from build123d import *

# Parameters (mm, degrees)
BOSS_EXTRUDE1_DEPTH = 5
SKETCH2_R           = 1.5
BOSS_EXTRUDE2_DEPTH = 7
SKETCH4_R           = 1
CUT_EXTRUDE1_DEPTH  = 21.732622043


with BuildPart() as part:
    # Sketch1 → Boss-Extrude1 (new body)
    with BuildSketch(Plane.XY):
        with BuildLine():
            ThreePointArc((12.735353306, 10.993667304), (8.407166921, 10.537476108), (5.016332041, 7.809189722))
            ThreePointArc((5.016332041, 7.809189722), (3.545099052, 3.440082341), (7.125107355, 6.34476242))
            ThreePointArc((7.125107355, 6.34476242), (9.612326684, 9.052857395), (12.735353306, 10.993667304))
        make_face()
    extrude(amount=BOSS_EXTRUDE1_DEPTH)

    # Sketch2 → Boss-Extrude2 (add)
    with BuildSketch(Plane.XY.offset(5)):
        with Locations((4.914048995, 5.411370258)):
            Circle(SKETCH2_R)
    extrude(amount=BOSS_EXTRUDE2_DEPTH)

    # Sketch4 → Cut-Extrude1 (cut, through all)
    with BuildSketch(Plane(origin=(0, 0, 0), x_dir=(-1, 0, 0), z_dir=(0, 0, -1))):
        with Locations((-6.764513076, 8.009147455)):
            Circle(SKETCH4_R)
    extrude(amount=-CUT_EXTRUDE1_DEPTH, mode=Mode.SUBTRACT)


solid = part.part
Part model, mm, in its own coordinate system. A direction names the side the tool comes from. Coordinates: 2 decimals unless noted, no trailing zeros. Order: outer loops, then holes, each group sorted by start corner. A loop starts at its lowest first (then second) coordinate and runs counter-clockwise, first axis right, second up. Notation, with made-up numbers: M -13,41 L 45,41 A34 cw 45,71 Z; hole C 14.25,82 d9. An arc over 180 degrees is marked long. Use a Markdown table: item, result.
(1) Pull direction Y, two halves, no side cores. Call faces 1 (the cylindrical face through (8.46, 10.56, 2.46)), 2 (the flat face through (6, 7, 0)), 3 (the cylindrical face through (6.303, 7.122, 2.465)): released by +Y, released by -Y, zero draft, split by the parting line, or undercut.
A:
| item | result |
|---|---|
| face 1 | released by +Y |
| face 2 | zero draft |
| face 3 | undercut |
(2) Probe L1, parallel to Z at x = 6.5, y = 6.5; L2, parallel to Y at x = 6, z = 3.5; L3, parallel to Y at x = 10, z = 2.5. List the from-to ranges inside material, lowest first.
A:
| item | result |
|---|---|
| L1 | z = 0 to 5 |
| L2 | y = 3.27 to 7.36, 8.65 to 8.96 |
| L3 | y = 9.36 to 11 |
(3) Cut at A-A on x = 7.5. Write the cut outline in (y, z).
A:
| item | result |
|---|---|
| outline | M 6.86,0 L 7.33,0 L 7.33,5 L 6.86,5 Z; M 8.69,0 L 10.09,0 L 10.09,5 L 8.69,5 Z |
(4) Cut at C-C on y = 5.75. Write the cut outline in (x, z).
A:
| item | result |
|---|---|
| outline | M 2.54,0 L 7.29,0 L 7.29,5 L 6.38,5 L 6.38,12 L 3.45,12 L 3.45,5 L 2.54,5 Z |
(5) Cut at D-D on z = 2. Write the cut outline in (x, y).
A:
| item | result |
|---|---|
| outline | M 5.02,7.81 A2.4 ccw long 7.13,6.34 A13.57 cw 12.74,10.99 A7.71 ccw Z; hole C 6.76,8.01 d2 |
(6) Flat gauge pins, fed straight in: pin 1 (6 mm diameter, centred on x = 4.5, z = 8.5, fed in from +Y); pin 2 (1.5 mm diameter, centred on x = 7, y = 7.5, fed in from -Z); pin 3 (1.8 mm diameter, centred on x = 6.76, y = 8.01, fed in from +Z); pin 4 (1.5 mm diameter, centred on x = 6, z = 9, fed in from -Y). Where does each tip first touch, or does it go through?
A:
| item | result |
|---|---|
| pin 1 | stops at y = 6.91 |
| pin 2 | stops at z = 0 |
| pin 3 | passes through |
| pin 4 | stops at y = 3.95 |
(7) Cut at B-B on y = 8.25. Write the cut outline in (x, z).
A:
| item | result |
|---|---|
| outline | M 5.35,0 L 5.79,0 L 5.79,5 L 5.35,5 Z; M 7.74,0 L 8.73,0 L 8.73,5 L 7.74,5 Z |
(8) Tool access for faces 4 (the cylindrical face through (5.72, 6.676, 8.451)), 5 (the cylindrical face through (3.475, 3.491, 2.465)): list every direction of +Z, -Z, +X, -X, +Y, -Y with a clear straight run to the whole face (end or side of a thin tool).
A:
| item | result |
|---|---|
| face 4 | +Z |
| face 5 | +Z, -Z |
